Geometry check sheet. Reference: drawing and pictorial views, mm from the part's lowest x, y, z. Round coordinates to 2 decimals unless told otherwise and drop trailing zeros. Write each loop counter-clockwise with the first axis right and the second up, starting at its lowest first coordinate (ties: lowest second). Pieces come first, ordered by that corner, then holes. Notation, with made-up numbers: (85.5, -19.75) -> (118.5, -19.75) arc R11 ccw to (118.5, -12.75) -> close; hole circle Ø8 at (38.25, 89.25). An arc over 180 degrees is marked (long way). Answer as a JSON object with one key per item and string values. Group by question number.
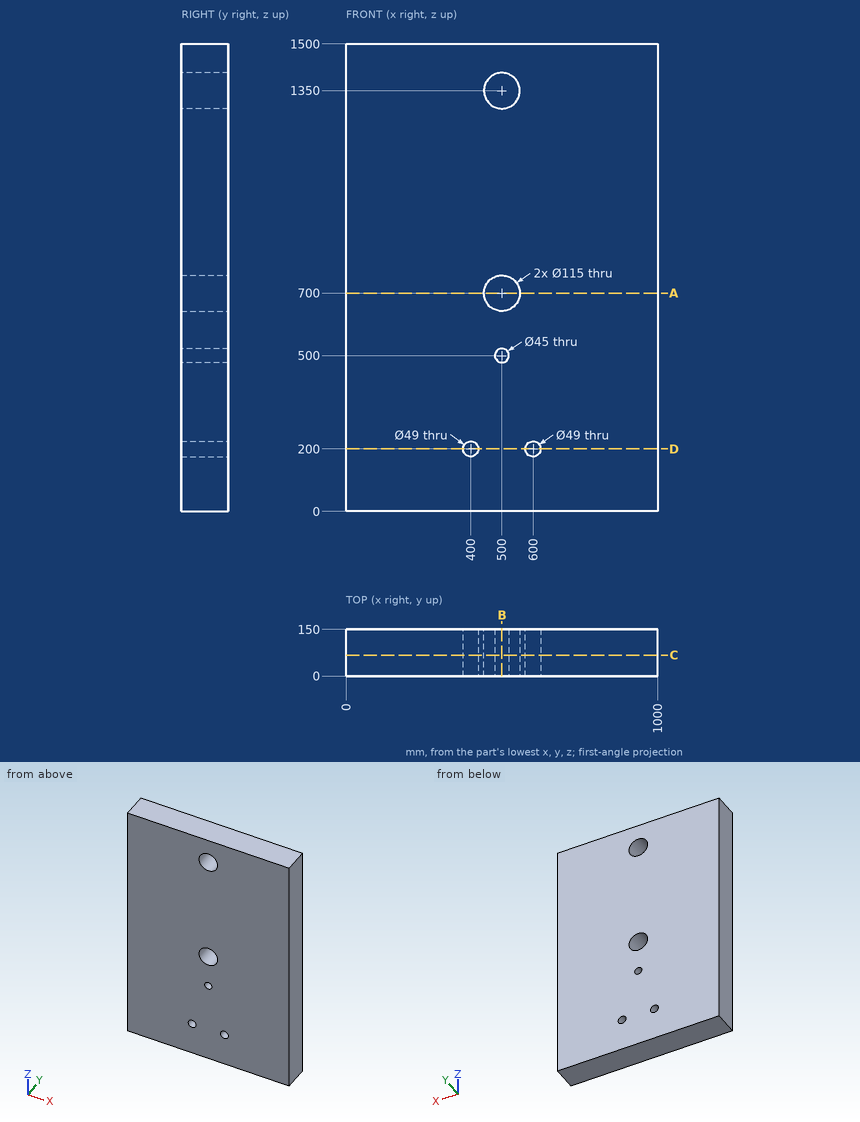
(1) Section check A-A on z = 700. Record the cut outline in (x, y).
(2) Go/stop test with a flat-tipped pin: pin 1 Ø4 at (y, z) = (126, 569.5) entering from -X. Record where the tip stops, or that it passes through.
(3) Scan lines: line 1 along Z through (x, y) = (600, 38); line 2 along X through (y, z) = (128, 1344); line 3 along Z through (x, y) = (500, 100). Record each from-to range of solid material in increasing order.
(4) Section check B-B on x = 500. Record the cut outline in (y, z), then the cut area to 3 significant figures.
(5) Section check D-D on z = 200. Record the cut outline in (x, y).
(6) Section check C-C on y = 67. Record the cut outline in (x, z), then the cut area to 3 significant figures.
Data:
{
 "1": {"outline": "(0, 0) -> (442.5, 0) -> (442.5, 150) -> (0, 150) -> close; (557.5, 0) -> (1000, 0) -> (1000, 150) -> (557.5, 150) -> close"},
 "2": {"pin 1": "stops at x = 0"},
 "3": {"line 1": "z = 0 to 175.5, 224.5 to 1500", "line 2": "x = 0 to 442.81, 557.19 to 1000", "line 3": "z = 0 to 477.5, 522.5 to 642.5, 757.5 to 1292.5, 1407.5 to 1500"},
 "4": {"outline": "(0, 0) -> (150, 0) -> (150, 477.5) -> (0, 477.5) -> close; (0, 522.5) -> (150, 522.5) -> (150, 642.5) -> (0, 642.5) -> close; (0, 757.5) -> (150, 757.5) -> (150, 1292.5) -> (0, 1292.5) -> close; (0, 1407.5) -> (150, 1407.5) -> (150, 1500) -> (0, 1500) -> close", "area": "184,000 mm²"},
 "5": {"outline": "(0, 0) -> (375.5, 0) -> (375.5, 150) -> (0, 150) -> close; (424.5, 0) -> (575.5, 0) -> (575.5, 150) -> (424.5, 150) -> close; (624.5, 0) -> (1000, 0) -> (1000, 150) -> (624.5, 150) -> close"},
 "6": {"outline": "(0, 0) -> (1000, 0) -> (1000, 1500) -> (0, 1500) -> close; hole circle Ø49 at (400, 200); hole circle Ø115 at (500, 700); hole circle Ø115 at (500, 1350); hole circle Ø45 at (500, 500); hole circle Ø49 at (600, 200)", "area": "1,470,000 mm²"}
}
